Autodesk Inventor part; units mm, degrees
ref_plane "YZ Plane" through (0, 0, 0) normal (1, 0, 0) x (0, 1, 0)
ref_plane "XZ Plane" through (0, 0, 0) normal (0, 1, 0) x (-1, 0, 0)
ref_plane "XY Plane" through (0, 0, 0) normal (0, 0, 1) x (1, 0, 0)
sketch "Sketch1" plane through (0, 0, 0) normal (0, 1, 0) x (-1, 0, 0)
  circle A0 centre (0, 0) radius 14.2875
  circle A1 centre (-98.1811, 12.7) radius 14.2875
  circle A2 centre (98.7952, -6.35) radius 14.2875
  circle A3 centre (98.7952, -6.35) radius 20.6375 construction
  circle A4 centre (0, 0) radius 20.6375 construction
  circle A5 centre (-98.1811, 12.7) radius 20.6375 construction
  circle A6 centre (67.0452, -6.35) radius 4.7625 construction
  circle A7 centre (-38.1, 0) radius 4.7625 construction
  circle A8 centre (67.0452, -6.35) radius 11.1125 construction
  circle A9 centre (-38.1, 0) radius 11.1125 construction
  line L0 (100.1189, 14.245) -> (1.3237, 20.595)
  line L1 (2.6475, 20.467) -> (-95.5336, 33.167)
  line L2 (-100.8285, -7.767) -> (-2.6475, -20.467)
  line L3 (97.4714, -26.945) -> (-1.3237, -20.595)
  arc A10 (-2.6475, -20.467) -> (-1.3237, -20.595) centre (0, 0) ccw
  arc A11 (97.4714, -26.945) -> (100.1189, 14.245) centre (98.7952, -6.35) ccw
  arc A12 (-95.5336, 33.167) -> (-100.8285, -7.767) centre (-98.1811, 12.7) ccw
  point P0 (1.9877, 20.5523)
  dimension "d0" = 28.575
  dimension "d1" = 98.999
  dimension "d2" = 98.999
  dimension "d3" = 12.7
  dimension "d4" = 6.35
  dimension "d5" = 6.35
  dimension "d6" = 6.35
  dimension "d7" = 6.35
  dimension "d8" = 31.75
  dimension "d9" = 38.1
  dimension "d10" = 9.525
  dimension "d11" = 6.35
extrude "Extrusion1" add sketch "Sketch1" along normal blind 6.35
hole "Hole1" at (38.1, 0, 0) at (-67.0452, 0, -6.35) direction (0, 1, 0) diameter 5.1054 end through all
properties part number "GP3-004" material "Aluminum 6061"
The model under review builds one solid part; all positions refer to its coordinate system, in mm. Round coordinates to 2 decimals unless told otherwise and drop trailing zeros. Order: outer loops, then holes, each group sorted by start corner. A loop starts at its lowest first (then second) coordinate and runs counter-clockwise, first axis right, second up. Notation, with made-up numbers: (65, -33) -> (102, -33) arc R26 cw to (102, 5) -> close; hole circle Ø3 at (-9.5, -34.75). An arc over 180 degrees is marked (long way). Use CSV: the item, a comma, the result in double quotes. Start each with the question number.
(1) Insertion check: pin 1 (1 mm diameter, centred on x = 63.5, y = 1.5, fed in from -Z); pin 2 (3 mm diameter, centred on y = 2.5, z = -2, fed in from +X); pin 3 (3 mm diameter, centred on x = 38.1, z = 0, fed in from -Y). Each pin has a flat end and moves straight along its axis. Give the tip position at first contact, or say it passes through.
(2) Consider section C-C on y = 4.25. State how many separate pieces and enclosed holes the cut face has, and give its area (3 significant figures).
(3) Consider section A-A on x = 38.1. Write out the cut boundary in (y, z).
(4) Wall thickness on probe 1 along X at (y, z) = (5.25, -3.5); probe 2 along X at (y, z) = (2.5, -6); probe 3 along Z at (x, y) = (4, 0.5): over which ranges is each line inside the solid? List them lowest first. Write a range as from..to.
(5) Mouldability with a two-part tool opening along Z and no side actions: class faces 1 (the face through (35.57, 3.22, 0.33)), 2 (the face through (-69.576, 3.219, -6.018)), 3 (the face through (1, 6.35, 17)), 4 (the face through (-51.74, 3.131, 17.354)) as pulls with the +Z half, pulls with the -Z half, needs draft (parallel to the pull), parting line crosses it, or undercut.
(6) Consider section B-B on z = 23. Write out the cut boundary in (x, y).
(7) Consider section D-D on z = -12. Write out the cut boundary in (x, y), and give its area (3 significant figures).
Responses:
1,pin 1,"z = -12.66"
1,pin 2,"x = 114.05"
1,pin 3,"through"
2,separate pieces,"1"
2,enclosed holes,"5"
2,area,"7,550 mm²"
3,outline,"(0, -15.88) -> (6.35, -15.88) -> (6.35, -2.55) -> (0, -2.55) -> close; (0, 2.55) -> (6.35, 2.55) -> (6.35, 25.74) -> (0, 25.74) -> close"
4,probe 1,"-119.23..-112.8, -84.79..-13.85, 13.85..110.97"
4,probe 2,"-119.43..-113.08, -84.51..-69.57, -64.52..-12.97, 12.97..106.91"
4,probe 3,"-20.29..-13.72, 13.72..21.33"
5,face 1,"undercut"
5,face 2,"undercut"
5,face 3,"needs draft"
5,face 4,"pulls with the +Z half"
6,outline,"(16.93, 0) -> (88.28, 0) -> (88.28, 6.35) -> (16.93, 6.35) -> close; (108.08, 0) -> (116.06, 0) -> (116.06, 6.35) -> (108.08, 6.35) -> close"
7,outline,"(-118.64, 0) -> (-111.92, 0) -> (-111.92, 6.35) -> (-118.64, 6.35) -> close; (-85.67, 0) -> (-7.75, 0) -> (-7.75, 6.35) -> (-85.67, 6.35) -> close; (7.75, 0) -> (68.1, 0) -> (68.1, 6.35) -> (7.75, 6.35) -> close"
7,area,"921 mm²"
